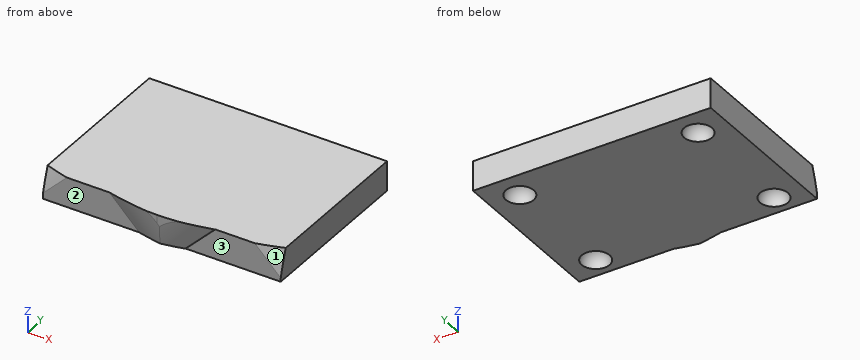
Autodesk Inventor part; units mm, degrees
ref_plane "Work Plane2" through (14.3627, 1.55, 6) normal (0, 0, 1) x (1, 0, 0)
ref_plane "Work Plane3" through (11.8127, 24, 6) normal (-1, 0, 0) x (0, 0, 1)
ref_plane "Work Plane4" through (26.8127, 23.9, 43.6151) normal (-0.7071068, 0, 0.7071068) x (-0.7071068, 0, -0.7071068)
ref_plane "Work Plane1" through (0, -12.9, 0) normal (0, 0, 1) x (1, 0, 0)
sketch "Sketch1" plane through (0, -12.9, 0) normal (0, 0, 1) x (1, 0, 0)
  circle A0 centre (26.8127, 14) radius 1.4 construction
  line L0 (6.8127, 27.5) -> (46.8127, 27.5)
  line L1 (46.8127, 27.5) -> (46.8127, 0.5)
  line L2 (46.8127, 0.5) -> (6.8127, 0.5)
  line L3 (6.8127, 0.5) -> (6.8127, 27.5)
  line L4 (6.8127, 27.5) -> (46.8127, 0.5) construction
  line L5 (46.8127, 27.5) -> (6.8127, 0.5) construction
  circle A1 centre (26.8127, 14) radius 12.7 construction
  circle A2 centre (26.8127, 14) radius 13
  line L6 (6.8127, 27.5) -> (46.8127, 27.5)
  line L7 (46.8127, 27.5) -> (46.8127, 28.5)
  line L8 (46.8127, 28.5) -> (6.8127, 28.5)
  line L9 (6.8127, 28.5) -> (6.8127, 27.5)
  point P0 (0, 12.9)
  dimension "d0" = 40
  dimension "d1" = 27
  dimension "d2" = 0.3
  dimension "d14" = 1
ref_plane "Work Plane2" through (14.3627, 1.55, 6) normal (0, 0, 1) x (1, 0, 0)
extrude "Extrusion1" add sketch "Sketch1" along normal up to surface (6 mm away)
ref_plane "Work Plane3" through (11.8127, 24, 6) normal (-1, 0, 0) x (0, 0, 1)
sketch "Sketch2" plane through (11.8127, 24, 6) normal (-1, 0, 0) x (0, 0, 1)
  line L0 (-9.3, 0) -> (1.55, 0)
  line L1 (-6, -35.9) -> (-6, -9.9)
  line L2 (-10.9, -34.4) -> (0.6933, -34.4)
  line L3 (-10.9, -31.4) -> (0.6933, -31.4)
  line L4 (-10.9, -14.4) -> (0.6933, -14.4)
  line L5 (-10.9, -11.4) -> (0.6933, -11.4)
  arc A0 (-5.3, -10.45) -> (-5.3, -15.35) centre (-5.3, -12.9) ccw
  arc A1 (-5.4335, -30.45) -> (-5.4335, -35.35) centre (-5.4335, -32.9) ccw
  line L6 (-5.4335, -35.35) -> (-5.4335, -30.45)
  line L7 (-5.3, -15.35) -> (-5.3, -10.45)
  point P0 (-6, -24)
  dimension "d22" = 4.9
  dimension "d23" = 1.5
  dimension "d24" = 1.5
revolve "Revolution1" cut sketch "Sketch2" angle 360 about axis through (11.8127, 8.65, 0.7) along (0, 1, 0) contours A0 L4 L1 | L1 L4 L7 A0 | L4 A0 L5 L1 | L1 L5 L7 L4 | L5 A0 L1 | L1 A0 L7 L5
pattern_linear "Rectangular Pattern1" count 2 spacing 20 along (0, -1, 0) count 2 spacing 30 along (1, 0, 0) of "Revolution1"
sketch "Sketch3" plane through (6.8127, -12.4, 6) normal (0, 0, 1) x (1, 0, 0)
  ellipse E0 centre (20, 24.3) end of major axis (41.0718, 24.3) minor radius 14.9 (7.3193, 12.4) -> (20, 9.4) ccw construction
  ellipse E1 centre (20, 24.3) end of major axis (41.0718, 24.3) minor radius 14.9 (20, 9.4) -> (32.6807, 12.4) ccw construction
  circle A0 centre (20, 13.5) radius 13 construction
  line L0 (40, 0) -> (0, 0) construction
  line L1 (40, 28) -> (40, 0) construction
  line L2 (0, 28) -> (40, 28) construction
  line L3 (0, 0) -> (0, 28) construction
  circle A1 centre (20, 13.5) radius 13 construction
  line L4 (40, 0) -> (0, 0)
  line L5 (10.0003, 0) -> (29.9997, 0)
  spline S0 degree 5 poles (2.3021, 2.9833) (5.5467, 1.2547) (9.0339, -0.0186) (12.6471, -0.8521) (16.3235, -1.2698) (20, -1.2699) knots 0 0 0 0 0 0 1 1 1 1 1 1
  spline S1 degree 5 poles (20, -1.2699) (23.6765, -1.2698) (27.3529, -0.8521) (30.9661, -0.0186) (34.4533, 1.2547) (37.6979, 2.9833) knots 0 0 0 0 0 0 1 1 1 1 1 1
  point P0 (-6.8127, 12.4)
extrude "Extrusion2" add sketch "Sketch3" against normal up to surface (6 mm away)
ref_plane "Work Plane4" through (26.8127, 23.9, 43.6151) normal (-0.7071068, 0, 0.7071068) x (-0.7071068, 0, -0.7071068)
sketch "Sketch4" plane through (26.8127, 23.9, 43.6151) normal (-0.7071068, 0, 0.7071068) x (-0.7071068, 0, -0.7071068)
  arc A0 (33.8666, 23.9) -> (15.9334, 23.9) centre (24.9, 12) ccw
  ellipse E0 centre (26.5979, 22.8) end of major axis (26.5979, 35.8) minor radius 9.1924 construction
  line L0 (12.4558, 36.3) -> (19.5271, 36.3) construction
  line L1 (12.4558, 8.3) -> (12.4558, 36.3) construction
  line L2 (40.74, 8.3) -> (12.4558, 8.3) construction
  line L3 (40.74, 36.3) -> (40.74, 8.3) construction
  line L4 (33.6687, 36.3) -> (40.74, 36.3)
  arc A1 (33.5545, 36.3) -> (9.1298, 32.4131) centre (24.9, 12) ccw
  line L5 (33.6687, 36.3) -> (40.74, 36.3)
  line L6 (33.5545, 36.3) -> (40.74, 36.3)
  line L7 (40.74, 36.3) -> (40.74, 42.5179)
  line L8 (40.74, 42.5179) -> (9.2813, 42.9694)
  line L9 (9.2813, 42.9694) -> (9.1298, 32.4131)
  point P0 (49.8, 23.9)
extrude "Extrusion3" cut sketch "Sketch4" against normal through all
ref_plane "Work Plane5" through (62.0266, 23.9, 8.4012) normal (0.7071068, 0, 0.7071068) x (-0.7071068, 0, 0.7071068)
sketch "Sketch5" plane through (62.0266, 23.9, 8.4012) normal (0.7071068, 0, 0.7071068) x (-0.7071068, 0, 0.7071068)
  arc A0 (33.8666, 23.9) -> (15.9334, 23.9) centre (24.9, 12) ccw
  arc A1 (40.4723, 32.6668) -> (9.3277, 32.6668) centre (24.9, 12) ccw
  line L0 (16.1313, 36.3) -> (11.8886, 36.3)
  line L1 (16.1313, 36.3) -> (16.2449, 36.3865) construction
  line L2 (16.2449, 36.3865) -> (16.1313, 36.3)
  line L3 (40.4723, 32.6668) -> (40.4723, 41.9024)
  line L4 (40.4723, 41.9024) -> (12.0732, 41.9024)
  line L5 (12.0732, 41.9024) -> (11.8886, 36.3)
  point P0 (37.9189, 23.9)
extrude "Extrusion4" cut sketch "Sketch5" against normal through all
sketch "Sketch6" plane through (6.8127, 15.6, 6) normal (0, 0, 1) x (1, 0, 0)
  circle A0 centre (20, -14.5) radius 13
  point P0 (-6.8127, -15.6)
extrude "Extrusion5" add sketch "Sketch6" against normal up to surface (6 mm away)
sketch "Sketch7" plane through (6.8127, 15.6, 0) normal (0, 1, 0) x (1, 0, 0)
  line L0 (0, -6) -> (40, -6) construction
  line L1 (40, 0) -> (40, -6) construction
  line L2 (40, 0) -> (0, 0) construction
  line L3 (0, 0) -> (0, -6) construction
  line L4 (0, -6) -> (40, -6)
  line L5 (40, -6) -> (40, -5)
  line L6 (40, -5) -> (0, -5)
  line L7 (0, -5) -> (0, -6)
  point P0 (-6.8127, 0)
  dimension "d27" = 1
extrude "Extrusion6" cut sketch "Sketch7" against normal through all
properties part number "20_Cube_Insert_Kinematic_Mirrormount_45_Thorlabsadapter"
Work out the finished part from the listing and answer in its coordinate system (mm). Face numbers are marked on the shaded views. A direction names the side the tool comes from. Coordinates: 2 decimals unless noted, no trailing zeros. Write each loop counter-clockwise with the first axis right and the second up, starting at its lowest first coordinate (ties: lowest second). Pieces come first, ordered by that corner, then holes.
1. The part is cut by section C-C, the plane x = 16.5. Write down the section's boundary in (y, z).
Results list:
outline: (-12.4, 0) - (15.6, 0) - (15.6, 5) - (-12.4, 5) - close
2. Consider line 1 along Y through (x, z) = (40.5, 1.35); line 2 along X through (y, z) = (11.25, 1.35); line 3 along Y through (x, z) = (13, 1.3). Determine where each line is inside the solid, lowest interval first.
Results list:
line 1: y = -12.4 to -10.86, -6.94 to 9.14, 13.06 to 15.6
line 2: x = 6.81 to 9.46, 14.17 to 39.46, 44.17 to 46.81
line 3: y = -12.4 to -10.96, -6.84 to 9.04, 13.16 to 15.6
3. The part is cut by section B-B, the plane z = 2.35. State how many separate pieces and enclosed holes the cut face has, and give its area (3 significant figures).
Results list:
separate pieces: 1
enclosed holes: 4
area: 1,090 mm2
4. The part is cut by section A-A, the plane x = 41. Write down the section's boundary in (y, z).
Results list:
outline: (-12.4, 0) - (-11.1, 0) arc R2.31 cw (long way) to (-6.7, 0) - (8.9, 0) arc R2.31 cw (long way) to (13.3, 0) - (15.6, 0) - (15.6, 5) - (-12.4, 5) - close
5. For the marked faces 1, 2 and 3, determine the directions among +Z, -Z, +X, -X, +Y, -Y from which every point of the face is accessible in a straight line to the end or side of a thin tool.
Results list:
face 1: +Z, +X, -Y
face 2: -Z, -X, -Y
face 3: -Z, +X, -Y
